Autodesk Inventor part; units mm, degrees
ref_plane "YZ Plane" through (0, 0, 0) normal (1, 0, 0) x (0, 1, 0)
ref_plane "XZ Plane" through (0, 0, 0) normal (0, 1, 0) x (-1, 0, 0)
ref_plane "XY Plane" through (0, 0, 0) normal (0, 0, 1) x (1, 0, 0)
sketch "Block1" plane through (0, 0, 0) normal (0, 0, 1) x (1, 0, 0)
  line L0 (0.22, -40.22) -> (-200.22, -40.22)
  line L1 (-200.22, -40.22) -> (-200.22, 0.22)
  line L2 (-200.22, 0.22) -> (0.22, 0.22)
  line L3 (0.22, 0.22) -> (0.22, -40.22)
  circle A0 centre (-5.9987, -35) radius 2.22
  circle A1 centre (-5.9987, -20) radius 2.22
  circle A2 centre (-5.9987, -5) radius 2.22
  circle A3 centre (-185, -25) radius 5.22
  circle A4 centre (-194.0013, -35) radius 2.22
  circle A5 centre (-194.0013, -5) radius 2.22
  circle A6 centre (-194.0013, -20) radius 2.22
  point P0 (-106.5385, -20.3846)
sketch "Sketch1" plane through (0, 0, 0) normal (0, 1, 0) x (-1, 0, 0)
  line L0 (0, 0) -> (200, 0)
  line L1 (200, 0) -> (200, 40)
  line L2 (200, 40) -> (0, 40)
  line L3 (0, 40) -> (0, 0)
  circle A0 centre (5.9987, 5) radius 2
  line L4 (5.9987, -4.5949) -> (5.9987, 47.4768)
  circle A1 centre (5.9987, 35) radius 2
  circle A2 centre (5.9987, 20) radius 2
  line L5 (100, 57.9252) -> (100, -15.7167)
  circle A3 centre (194.0013, 5) radius 2
  circle A4 centre (194.0013, 35) radius 2
  circle A5 centre (194.0013, 20) radius 2
  circle A6 centre (185, 25) radius 5
  dimension "d0" = 200
  dimension "d1" = 40
  dimension "d4" = 4
  dimension "d5" = 4
  dimension "d6" = 5
  dimension "d7" = 5
  dimension "d8" = 4
  dimension "d9" = 20
  dimension "d10" = 100
  dimension "d13" = 10
  dimension "d14" = 15
  dimension "d15" = 15
extrude "Extrusion3" add sketch "Sketch1" along normal blind 10 contours L3 L2 L4 A1 A2 A0 L0 | L4 A0 A2 A1 L2 L5 L0 | L5 L2 L1 L0
sketch "Sketch2" plane through (0, 10, 0) normal (0, 1, 0) x (1, 0, 0)
  circle A0 centre (-185, -25) radius 5
  circle A1 centre (-194.0013, -20) radius 2
  circle A2 centre (-194.0013, -35) radius 2
  circle A3 centre (-194.0013, -5) radius 2
  circle A4 centre (-5.9987, -20) radius 2
  circle A5 centre (-5.9987, -35) radius 2
  circle A6 centre (-5.9987, -5) radius 2
  line L0 (0, 0) -> (-200, 0)
  line L1 (-200, 0) -> (-200, -40)
  line L2 (-200, -40) -> (0, -40)
  line L3 (0, -40) -> (0, 0)
sketch "DXF" plane through (0, 0, 0) normal (0, 1, 0) x (-1, 0, 0)
  point P0 (0, 0)
properties part number "gripsupport"
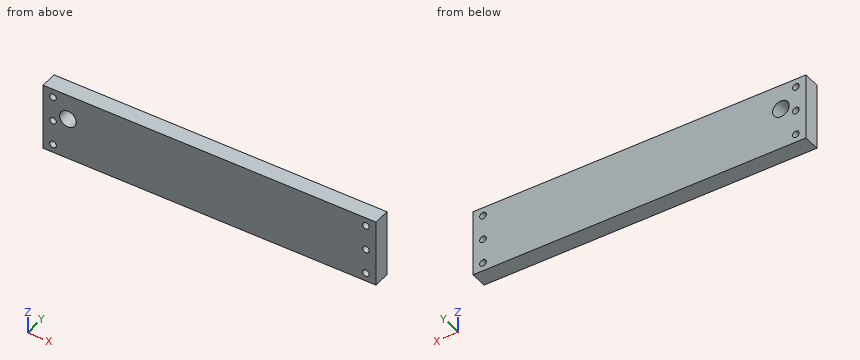
Model file for the job. Use its own axes, mm. Give positions to 0.01 mm unless a question says otherwise; leave off trailing zeros. Order: outer loops, then holes, each group sorted by start corner. A loop starts at its lowest first (then second) coordinate and runs counter-clockwise, first axis right, second up. Notation, with made-up numbers: (-17, 20.5) - (-5, 20.5) arc R13 ccw to (-5, 42.5) - close; hole circle Ø1 at (59.25, 89). An arc over 180 degrees is marked (long way). Write item = value, one per line. Start each with the question number.
1. Cut at B-B, the plane y = 5.75. List the corners of the cut face in (x, z).
2. Cut at C-C, the plane z = 5. List the corners of the cut face in (x, y).
3. Cut at A-A, the plane z = 25. List the corners of the cut face in (x, y).
4. Drop a flat-ended pin along its axis: P1, Ø6, axis at x = -79.5, y = 2.5, coming from the -Z side. Give the stop position or say it passes through.
5. Probe line 1 along Z through (x, y) = (-185, 3.25); line 2 along X through (y, z) = (5.25, 36); line 3 along X through (y, z) = (5.5, 28). List the from-to ranges inside material, lowest first.
Taken from the geometry:
q1.outline = (-200, 0) - (0, 0) - (0, 40) - (-200, 40) - close; hole circle Ø4 at (-194, 5); hole circle Ø4 at (-194, 20); hole circle Ø4 at (-194, 35); hole circle Ø10 at (-185, 25); hole circle Ø4 at (-6, 5); hole circle Ø4 at (-6, 20); hole circle Ø4 at (-6, 35)
q2.outline = (-200, 0) - (-196, 0) - (-196, 10) - (-200, 10) - close; (-192, 0) - (-8, 0) - (-8, 10) - (-192, 10) - close; (-4, 0) - (0, 0) - (0, 10) - (-4, 10) - close
q3.outline = (-200, 0) - (-190, 0) - (-190, 10) - (-200, 10) - close; (-180, 0) - (0, 0) - (0, 10) - (-180, 10) - close
q4.P1 = 0
q5.line_1 = 0 to 20, 30 to 40
q5.line_2 = -200 to -195.73, -192.27 to -7.73, -4.27 to 0
q5.line_3 = -200 to -189, -181 to 0
